The model under review builds one solid part; all positions refer to its coordinate system, in mm. Round coordinates to 2 decimals unless told otherwise and drop trailing zeros. Order: outer loops, then holes, each group sorted by start corner. A loop starts at its lowest first (then second) coordinate and runs counter-clockwise, first axis right, second up.
1) Consider section C-C (z = -7). Give the boundary of the cut face in (x, y), then the cut area to 3 significant figures.
2) To check wall thickness, follow L1, parallel to X at y = 0.6, z = 7; L2, parallel to X at y = 0.45, z = 8; L3, parallel to X at y = 0.9, z = -0.5. State the ranges of each line that lie inside material, in increasing order.
3) Consider section B-B (z = 0). Give the boundary of the cut face in (x, y), then the cut area to 3 significant figures.
4) Consider section A-A (x = -7). Give the boundary of the cut face in (y, z), then the cut area to 3 significant figures.
5) Consider section D-D (x = 12.5). Give the boundary of the cut face in (y, z).
6) Mouldability with a two-part tool opening along X and no side actions: class faces 1 (the face through (0, 1, 12.5)), 2 (the face through (5.536, 0.986, -0.325)), 3 (the face through (27.5, 1, 0)), 4 (the face through (-20.06, 0.99, -0.33)) as pulls with the +X half, pulls with the -X half, needs draft (parallel to the pull), parting line crosses it, or undercut.
from build123d import *

# Parameters (mm, degrees)
SKETCH_1_W      = 55
SKETCH_1_H      = 25
SKETCH_1_R      = 1.5
SKETCH_1_R_2    = 4
EXTRUDE_1_DEPTH = 2


with BuildPart() as part:
    # 草图1 → 凸台-拉伸1 (new body)
    with BuildSketch(Plane(origin=(0, 0, 0), x_dir=(1, 0, 0), z_dir=(0, 1, 0))):
        Rectangle(SKETCH_1_W, SKETCH_1_H)
        with Locations(Location((0, 7, 0), (0, 0, 270))):
            Circle(SKETCH_1_R, mode=Mode.SUBTRACT)
        with Locations(Location((7, 0, 0), (0, 0, 270))):
            Circle(SKETCH_1_R, mode=Mode.SUBTRACT)
        with Locations(Location((0, -7, 0), (0, 0, 270))):
            Circle(SKETCH_1_R, mode=Mode.SUBTRACT)
        with Locations(Location((-7, 0, 0), (0, 0, 270))):
            Circle(SKETCH_1_R, mode=Mode.SUBTRACT)
        with Locations(Location((-18.598687937, 0, 0), (0, 0, 270))):
            Circle(SKETCH_1_R, mode=Mode.SUBTRACT)
        with Locations(Location((0, 0, 0), (0, 0, 270))):
            Circle(SKETCH_1_R_2, mode=Mode.SUBTRACT)
        with Locations(Location((18.795941944, 0, 0), (0, 0, 270))):
            Circle(SKETCH_1_R, mode=Mode.SUBTRACT)
        with Locations(Location((12.5, 7, 0), (0, 0, 270))):
            Circle(SKETCH_1_R, mode=Mode.SUBTRACT)
        with Locations(Location((12.5, -7, 0), (0, 0, 90))):
            Circle(SKETCH_1_R, mode=Mode.SUBTRACT)
        with Locations(Location((-12.5, -7, 0), (0, 0, 270))):
            Circle(SKETCH_1_R, mode=Mode.SUBTRACT)
        with Locations(Location((-12.5, 7, 0), (0, 0, 90))):
            Circle(SKETCH_1_R, mode=Mode.SUBTRACT)
    extrude(amount=EXTRUDE_1_DEPTH)


solid = part.part
Answer below:
1. outline: (-27.5, 0) - (-14, 0) - (-14, 2) - (-27.5, 2) - close; (-11, 0) - (-1.5, 0) - (-1.5, 2) - (-11, 2) - close; (1.5, 0) - (11, 0) - (11, 2) - (1.5, 2) - close; (14, 0) - (27.5, 0) - (27.5, 2) - (14, 2) - close
1. area: 92.0 mm2
2. L1: x = -27.5 to -14, -11 to -1.5, 1.5 to 11, 14 to 27.5
2. L2: x = -27.5 to -13.62, -11.38 to -1.12, 1.12 to 11.38, 13.62 to 27.5
2. L3: x = -27.5 to -20.01, -17.18 to -8.41, -5.59 to -3.97, 3.97 to 5.59, 8.41 to 17.38, 20.21 to 27.5
3. outline: (-27.5, 0) - (-20.1, 0) - (-20.1, 2) - (-27.5, 2) - close; (-17.1, 0) - (-8.5, 0) - (-8.5, 2) - (-17.1, 2) - close; (-5.5, 0) - (-4, 0) - (-4, 2) - (-5.5, 2) - close; (4, 0) - (5.5, 0) - (5.5, 2) - (4, 2) - close; (8.5, 0) - (17.3, 0) - (17.3, 2) - (8.5, 2) - close; (20.3, 0) - (27.5, 0) - (27.5, 2) - (20.3, 2) - close
3. area: 70.0 mm2
4. outline: (0, -12.5) - (2, -12.5) - (2, -1.5) - (0, -1.5) - close; (0, 1.5) - (2, 1.5) - (2, 12.5) - (0, 12.5) - close
4. area: 44.0 mm2
5. outline: (0, -12.5) - (2, -12.5) - (2, -8.5) - (0, -8.5) - close; (0, -5.5) - (2, -5.5) - (2, 5.5) - (0, 5.5) - close; (0, 8.5) - (2, 8.5) - (2, 12.5) - (0, 12.5) - close
6. face 1: needs draft
6. face 2: undercut
6. face 3: pulls with the +X half
6. face 4: undercut
